Model file for the job. Use its own axes, mm. Face numbers are marked on the shaded views. A direction names the side the tool comes from. Give positions to 0.01 mm unless a question says otherwise; leave off trailing zeros. Loops run counter-clockwise (first coordinate to the right, second up) from the corner with the lowest first, then second, coordinate; pieces in that order, holes last. Notation, with made-up numbers: (46.5, 85) - (74.5, 85) arc R15 cw to (74.5, 103) - close; hole circle Ø4 at (56, 65). An arc over 180 degrees is marked (long way). Use a Markdown table: item, result.
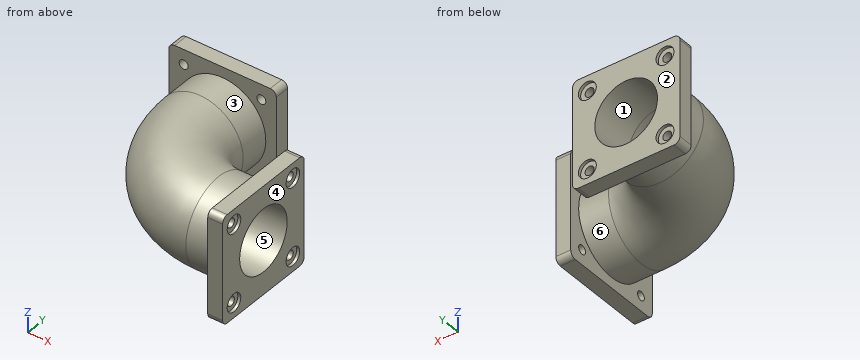
from build123d import *

# Parameters (mm, degrees)
SKETCH2_R           = 145
SKETCH2_R_2         = 105
SKETCH3_W           = 360
SKETCH3_H           = 360
SKETCH3_R           = 145
BOSS_EXTRUDE1_DEPTH = 50
FILLET1_R           = 20
SKETCH4_W           = 360
SKETCH4_H           = 360
SKETCH4_R           = 145
BOSS_EXTRUDE2_DEPTH = 50
FILLET2_R           = 20
SKETCH5_R           = 30
CUT_EXTRUDE1_DEPTH  = 10
SKETCH6_R           = 15
CUT_EXTRUDE2_DEPTH  = 40
CIRPATTERN1_COUNT   = 4
SKETCH7_R           = 30
CUT_EXTRUDE3_DEPTH  = 10
SKETCH8_R           = 15
CUT_EXTRUDE4_DEPTH  = 40
CIRPATTERN2_COUNT   = 4


with BuildPart() as part:
    # Sweep-Thin1: sweep along a path in Sketch1
    with BuildLine(Plane.XY) as sweep_thin1_path:
        Line((0, 0), (-150, 0))
        ThreePointArc((-150, 0), (-333.847763109, 76.152236891), (-410, 260))
        Line((-410, 260), (-410, 410))
    # Sketch2 → Sweep-Thin1 (sweep)
    with BuildSketch(Plane(origin=(0, 0, 0), x_dir=(0, 0, -1), z_dir=(1, 0, 0))):
        Circle(SKETCH2_R)
        Circle(SKETCH2_R_2, mode=Mode.SUBTRACT)
    sweep(path=sweep_thin1_path.line)

    # Sketch3 → Boss-Extrude1 (add)
    with BuildSketch(Plane(origin=(0, 0, 0), x_dir=(0, 0, -1), z_dir=(1, 0, 0))):
        Rectangle(SKETCH3_W, SKETCH3_H)
        Circle(SKETCH3_R, mode=Mode.SUBTRACT)
    extrude(amount=-BOSS_EXTRUDE1_DEPTH)

    # Fillet1
    fillet1_edges = [part.edges().sort_by_distance(p)[0] for p in [
        (-25, 180, -180),
        (-25, -180, -180),
        (-25, -180, 180),
        (-25, 180, 180),
    ]]
    fillet(fillet1_edges, radius=FILLET1_R)

    # Sketch4 → Boss-Extrude2 (add)
    with BuildSketch(Plane(origin=(0, 410, 0), x_dir=(1, 0, 0), z_dir=(0, 1, 0))):
        with Locations((-410, 0)):
            Rectangle(SKETCH4_W, SKETCH4_H)
        with Locations((-410, 0)):
            Circle(SKETCH4_R, mode=Mode.SUBTRACT)
    extrude(amount=-BOSS_EXTRUDE2_DEPTH)

    # Fillet2
    fillet2_edges = [part.edges().sort_by_distance(p)[0] for p in [
        (-590, 385, 180),
        (-590, 385, -180),
        (-230, 385, -180),
        (-230, 385, 180),
    ]]
    fillet(fillet2_edges, radius=FILLET2_R)

    # Sketch5 → Cut-Extrude1 (cut)
    with BuildSketch(Plane(origin=(0, 410, 0), x_dir=(1, 0, 0), z_dir=(0, 1, 0))):
        with Locations((-280, 130)):
            Circle(SKETCH5_R)
    cut_extrude1 = extrude(amount=-CUT_EXTRUDE1_DEPTH, mode=Mode.SUBTRACT)

    # Sketch6 → Cut-Extrude2 (cut)
    with BuildSketch(Plane(origin=(0, 400, 0), x_dir=(1, 0, 0), z_dir=(0, 1, 0))):
        with Locations((-280, 130)):
            Circle(SKETCH6_R)
    cut_extrude2 = extrude(amount=-CUT_EXTRUDE2_DEPTH, mode=Mode.SUBTRACT)

    # CirPattern1: Cut-Extrude1, Cut-Extrude2 ×4 about axis
    cirpattern1_axis = Axis((-410, 0, 0), (0, 1, 0))
    for i in range(1, CIRPATTERN1_COUNT):
        add(cut_extrude1.rotate(cirpattern1_axis, i * 360 / CIRPATTERN1_COUNT), mode=Mode.SUBTRACT)
        add(cut_extrude2.rotate(cirpattern1_axis, i * 360 / CIRPATTERN1_COUNT), mode=Mode.SUBTRACT)

    # Sketch7 → Cut-Extrude3 (cut)
    with BuildSketch(Plane(origin=(0, 0, 0), x_dir=(0, 0, -1), z_dir=(1, 0, 0))):
        with Locations((130, 130)):
            Circle(SKETCH7_R)
    cut_extrude3 = extrude(amount=-CUT_EXTRUDE3_DEPTH, mode=Mode.SUBTRACT)

    # Sketch8 → Cut-Extrude4 (cut)
    with BuildSketch(Plane(origin=(-10, 0, 0), x_dir=(0, 0, -1), z_dir=(1, 0, 0))):
        with Locations((130, 130)):
            Circle(SKETCH8_R)
    cut_extrude4 = extrude(amount=-CUT_EXTRUDE4_DEPTH, mode=Mode.SUBTRACT)

    # CirPattern2: Cut-Extrude3, Cut-Extrude4 ×4 about axis
    cirpattern2_axis = Axis((0, 0, 0), (1, 0, 0))
    for i in range(1, CIRPATTERN2_COUNT):
        add(cut_extrude3.rotate(cirpattern2_axis, i * 360 / CIRPATTERN2_COUNT), mode=Mode.SUBTRACT)
        add(cut_extrude4.rotate(cirpattern2_axis, i * 360 / CIRPATTERN2_COUNT), mode=Mode.SUBTRACT)


solid = part.part
(1) Mould opens along X. For the marked faces 1, 2 and 3 say: pulls with the +X half, pulls with the -X half, needs draft (parallel to the pull), parting line crosses it, or undercut.
Computed:
| item | result |
|---|---|
| face 1 | undercut |
| face 2 | needs draft |
| face 3 | parting line crosses it |
(2) Pin check, flat tips, straight feed: P1, Ø12, axis at y = 80.5, z = 65.5, coming from the +X side; P2, Ø18, axis at x = -292, z = 117, coming from the +Y side; P3, Ø2, axis at y = 44, z = 62.5, coming from the +X side; P4, Ø24, axis at x = -280, z = 130, coming from the -Y side. Stop position of each tip, or through.
Computed:
| item | result |
|---|---|
| P1 | x = 0 |
| P2 | y = 400 |
| P3 | x = -416.95 |
| P4 | y = -59.41 |
(3) Slice it at A-A, the plane z = 0. Write the cut outline in (x, y).
Computed:
| item | result |
|---|---|
| outline | (-590, 360) - (-555, 360) - (-555, 260) arc R405 ccw to (-150, -145) - (-50, -145) - (-50, -180) - (0, -180) - (0, -105) - (-150, -105) arc R365 cw to (-515, 260) - (-515, 410) - (-590, 410) - close; (-305, 260) arc R155 ccw to (-150, 105) - (0, 105) - (0, 180) - (-50, 180) - (-50, 145) - (-150, 145) arc R115 cw to (-265, 260) - (-265, 360) - (-230, 360) - (-230, 410) - (-305, 410) - close |
(4) Drill centre lines: probe 1 along Z at (x, y) = (-540, 402.75); probe 2 along Z at (x, y) = (-540, 368); probe 3 along Y at (x, z) = (-428.5, -162.5). Where is each one in solid material? Low to high. Write a range as [from, to].
Computed:
| item | result |
|---|---|
| probe 1 | [-180, -160], [-100, 100], [160, 180] |
| probe 2 | [-180, -145], [-115, 115], [145, 180] |
| probe 3 | [360, 410] |
(5) Slice it at C-C, the plane y = 336.5. Write the cut outline in (x, z).
Computed:
| item | result |
|---|---|
| outline | circle Ø290 at (-410, 0); hole circle Ø210 at (-410, 0) |
(6) Slice it at B-B, the plane x = -280. Count the separate pieces of the cut face and the enclosed holes in it, plus the area to 3 significant figures.
Computed:
| item | result |
|---|---|
| separate pieces | 3 |
| enclosed holes | 1 |
| area | 71,600 mm² |
(7) 3-axis set-ups, long thin cutter, end or side, ignore diameter. For the marked faces 4, 5 and 6: which of +Z, -Z, +X, -X, +Y, -Y reach the whole face in a straight line?
Computed:
| item | result |
|---|---|
| face 4 | +Z, -Z, +X, +Y, -Y |
| face 5 | +X |
| face 6 | none |
